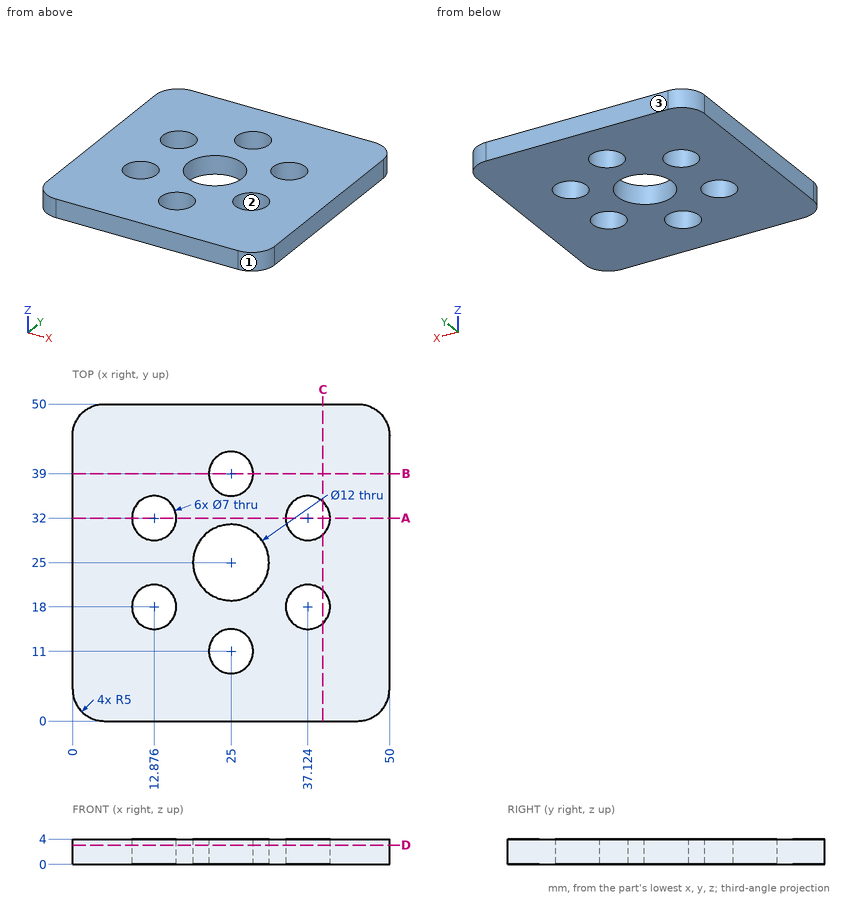
Verification items for this drawing (mm, ordinates from the low corner). Coordinates: 2 decimals unless noted, no trailing zeros. Loops run counter-clockwise (first coordinate to the right, second up) from the corner with the lowest first, then second, coordinate; pieces in that order, holes last. Notation, with made-up numbers: (-17.5, 13.25) - (-12.5, 13.25) arc R21 ccw to (-12.5, 17.25) - close; hole circle Ø8 at (71, -16.75). An arc over 180 degrees is marked (long way). Answer as a JSON object with one key per item and string values.
(1) Cross-section at D-D, the plane z = 3.05. Record the boundary of the cut face in (x, y) (1 decimal).
Response:
{"outline": "(0, 5) arc R5 ccw to (5, 0) - (45, 0) arc R5 ccw to (50, 5) - (50, 45) arc R5 ccw to (45, 50) - (5, 50) arc R5 ccw to (0, 45) - close; hole circle Ø7 at (12.9, 18); hole circle Ø7 at (12.9, 32); hole circle Ø12 at (25, 25); hole circle Ø7 at (25, 11); hole circle Ø7 at (25, 39); hole circle Ø7 at (37.1, 18); hole circle Ø7 at (37.1, 32)"}
(2) Cross-section at B-B, the plane y = 39. Record the boundary of the cut face in (x, z).
Response:
{"outline": "(0, 0) - (21.5, 0) - (21.5, 4) - (0, 4) - close; (28.5, 0) - (50, 0) - (50, 4) - (28.5, 4) - close"}
(3) Cross-section at A-A, the plane y = 32. Record the boundary of the cut face in (x, z) (1 decimal).
Response:
{"outline": "(0, 0) - (9.4, 0) - (9.4, 4) - (0, 4) - close; (16.4, 0) - (33.6, 0) - (33.6, 4) - (16.4, 4) - close; (40.6, 0) - (50, 0) - (50, 4) - (40.6, 4) - close"}
(4) Go/stop test with a flat-tipped pin: pin 1 Ø8 at (x, y) = (25, 39) entering from -Z. Record where the tip stops, or that it passes through.
Response:
{"pin 1": "stops at z = 0"}
(5) Cross-section at C-C, the plane x = 39.5. Record the boundary of the cut face in (y, z).
Response:
{"outline": "(0, 0) - (15.43, 0) - (15.43, 4) - (0, 4) - close; (20.57, 0) - (29.43, 0) - (29.43, 4) - (20.57, 4) - close; (34.57, 0) - (50, 0) - (50, 4) - (34.57, 4) - close"}
(6) Scan lines: line 1 along Y through (x, z) = (25, 1.65); line 2 along Y through (x, z) = (15, 2.9); line 3 along Y through (x, z) = (23.5, 2.9). Record each from-to range of solid material in increasing order.
Response:
{"line 1": "y = 0 to 7.5, 14.5 to 19, 31 to 35.5, 42.5 to 50", "line 2": "y = 0 to 15.22, 20.78 to 29.22, 34.78 to 50", "line 3": "y = 0 to 7.84, 14.16 to 19.19, 30.81 to 35.84, 42.16 to 50"}
(7) Mould release check, pull along X, two halves, no side actions. Record for the marked faces 1, 2 and 3: pulls with the +X half, pulls with the -X half, needs draft (parallel to the pull), parting line crosses it, or undercut.
Response:
{"face 1": "pulls with the +X half", "face 2": "undercut", "face 3": "needs draft"}
